```python
from build123d import *

# Parameters (mm, degrees)
F0_W      = 2
F0_H      = 60
F1_DEPTH  = 46
F2_DEPTH  = 2
F3_W      = 60
F3_H      = 3
F4_DEPTH  = 20
F5_W      = 60
F5_H      = 3
F6_DEPTH  = 20
F7_W      = 60
F7_H      = 46
F8_DEPTH  = 3
F10_DEPTH = 3


with BuildPart() as f1:
    # F0 (on Top) → F1 (new body)
    with BuildSketch(Plane.XY):
        with Locations((1, 30)):
            Rectangle(F0_W, F0_H)
    extrude(amount=F1_DEPTH)



with BuildPart() as f1b:
    # F0 (on Top) → F1, piece 2 (new body)
    with BuildSketch(Plane.XY):
        with Locations((59, 30)):
            Rectangle(F0_W, F0_H)
    extrude(amount=F1_DEPTH)


with BuildPart() as f1_1:
    add(f1.part)

    add(f1b.part)  # F2 merges F1b
    # F0 (on Top) → F2 (join)
    with BuildSketch(Plane.XY):
        with Locations((1, 30)):
            Rectangle(F0_W, F0_H)
        Polygon((2, 60), (2, 0), (4.7754659317, 0), (58, 0), (58, 60), align=None)
        with Locations((59, 30)):
            Rectangle(F0_W, F0_H)
    extrude(amount=F2_DEPTH)

    # F3 (on face) → F4 (join)
    with BuildSketch(Plane(origin=(0, 0, 0), x_dir=(0, -1, 0), z_dir=(-1, 0, 0))):
        with Locations((-30, 44.5)):
            Rectangle(F3_W, F3_H)
    extrude(amount=F4_DEPTH)

    # F5 (on face) → F6 (join)
    with BuildSketch(Plane.YZ.offset(60)):
        with Locations((30, 44.5)):
            Rectangle(F5_W, F5_H)
    extrude(amount=F6_DEPTH)

    # F7 (on face) → F8 (join)
    with BuildSketch(Plane(origin=(0, 60, 0), x_dir=(-1, 0, 0), z_dir=(0, 1, 0))):
        with Locations((-30, 23)):
            Rectangle(F7_W, F7_H)
    extrude(amount=-F8_DEPTH)

    # F9 (on face) → F10 (cut)
    with BuildSketch(Plane(origin=(0, 60, 0), x_dir=(-1, 0, 0), z_dir=(0, 1, 0))):
        with BuildLine():
            Line((-18.001411375, 46), (-18.001411375, 24.000384872))
            ThreePointArc((-18.001411375, 24.000384872), (-12.001411375, 18.000384872), (-6.001411375, 24.000384872))
            Line((-6.001411375, 24.000384872), (-6.001411375, 46))
            Line((-6.001411375, 46), (-18.001411375, 46))
        make_face()
        with BuildLine():
            Line((-42, 24), (-42, 46))
            Line((-42, 46), (-54, 46))
            Line((-54, 46), (-54, 24))
            ThreePointArc((-54, 24), (-48, 18), (-42, 24))
        make_face()
    extrude(amount=-F10_DEPTH, mode=Mode.SUBTRACT)


solid = f1_1.part
```
Here's how the part is built. I have some questions about the finished solid (model axes, mm). A direction names the side the tool comes from. Round coordinates to 2 decimals unless told otherwise and drop trailing zeros. Loops run counter-clockwise (first coordinate to the right, second up) from the corner with the lowest first, then second, coordinate; pieces in that order, holes last. Notation, with made-up numbers: (-17, 26.5) -> (11, 26.5) arc R5 ccw to (11, 30.5) -> close; hole circle Ø8 at (-36, 13.5). An arc over 180 degrees is marked (long way). Answer as CSV lines item,"result". Start each with the question number.
1. I'm going to push flat-ended pins straight in: P1, Ø13, axis at y = 31.5, z = 34, coming from the +X side; P2, Ø1, axis at x = 19, z = 33, coming from the -Y side; P3, Ø5, axis at y = 34.5, z = 13, coming from the -X side. Where does each tip first touch, or does it pass through?
2. For faces 5 (the face through (6.001, 59, 35)), 6 (the face through (70, 30, 43)), 7 (the face through (30, 29, 2)), which set-ups out of +Z, -Z, +X, -X, +Y, -Y let a thin tool reach every point of the face, with its end or its side?
3. Imagine slicing it at D-D on x = 48. Write out the boundary of the cut face in (y, z), plus the area to 3 significant figures.
4. Imagine slicing it at B-B on y = 32.5. Write out the boundary of the cut face in (x, z), plus the area to 3 significant figures.
5. Imagine slicing it at C-C on x = 20.5. Write out the boundary of the cut face in (y, z), plus the area to 3 significant figures.
6. Imagine slicing it at A-A on z = 29.5. Write out the boundary of the cut face in (x, y).
7. I need wall thicknesses on probe 1 along X at (y, z) = (22, 3.5); probe 2 along X at (y, z) = (40, 44); probe 3 along Z at (x, y) = (10, 50.5). Which ranges of each line are inside material? Lowest first, please. Write a range as from..to.
8. If we mould it in two halves opening along X, with no side actions, what happens to faces 1 (the face through (30, 30, 0)), 2 (the face through (18.001, 59, 35)), 3 (the face through (2, 28, 24)), 4 (the face through (0, 30, 21))? For each: pulls with the +X half, pulls with the -X half, needs draft (parallel to the pull), parting line crosses it, or undercut.
Solution:
1,P1,"x = 60"
1,P2,"y = 57"
1,P3,"x = 0"
2,face 5,"+Z, +Y, -Y"
2,face 6,"-Z, +X, +Y, -Y"
2,face 7,"+Z, -Y"
3,outline,"(0, 0) -> (60, 0) -> (60, 18) -> (57, 18) -> (57, 2) -> (0, 2) -> close"
3,area,"168 mm²"
4,outline,"(-20, 43) -> (0, 43) -> (0, 0) -> (60, 0) -> (60, 43) -> (80, 43) -> (80, 46) -> (58, 46) -> (58, 2) -> (2, 2) -> (2, 46) -> (-20, 46) -> close"
4,area,"416 mm²"
5,outline,"(0, 0) -> (60, 0) -> (60, 46) -> (57, 46) -> (57, 2) -> (0, 2) -> close"
5,area,"252 mm²"
6,outline,"(0, 0) -> (2, 0) -> (2, 57) -> (6, 57) -> (6, 60) -> (0, 60) -> close; (18, 57) -> (42, 57) -> (42, 60) -> (18, 60) -> close; (54, 57) -> (58, 57) -> (58, 0) -> (60, 0) -> (60, 60) -> (54, 60) -> close"
7,probe 1,"0..2, 58..60"
7,probe 2,"-20..2, 58..80"
7,probe 3,"0..2"
8,face 1,"needs draft"
8,face 2,"undercut"
8,face 3,"undercut"
8,face 4,"pulls with the -X half"
